```python
from build123d import *

# Parameters (mm, degrees)
F2_DEPTH = 2
F0_R     = 5
F3_DEPTH = 8


with BuildPart() as f2:
    # F1 (on Top) → F2 (new body)
    with BuildSketch(Plane.XY):
        with BuildLine():
            ThreePointArc((13.3352901354, 8.8413820755), (12.5684052501, -9.9012721137), (-5.473909682, -15.0345040754))
            ThreePointArc((-5.473909682, -15.0345040754), (-8.2417855801, -14.8458488198), (-10.6841578939, -16.1617307572))
            ThreePointArc((-10.6841578939, -16.1617307572), (-6.49143908, -46.9599083827), (21.8114936554, -34.112705003))
            Line((21.8114936554, -34.112705003), (25.1481622756, -18.7513405658))
            ThreePointArc((25.1481622756, -18.7513405658), (25.3446435428, -18.0783456566), (25.6333270757, -17.4394490656))
            ThreePointArc((25.6333270757, -17.4394490656), (27.3258914034, -0.6237467424), (16.5919494859, 12.4305670861))
            ThreePointArc((16.5919494859, 12.4305670861), (13.5674787289, 11.902767988), (13.3352901354, 8.8413820755))
        make_face()
    extrude(amount=-F2_DEPTH)

    # F0 (on Top) → F3 (join)
    with BuildSketch(Plane.XY):
        with BuildLine():
            ThreePointArc((9.3589739054, -12.9772727273), (2.1980630587, -15.8482970312), (-5.473909682, -15.0345040754))
            ThreePointArc((-5.473909682, -15.0345040754), (-8.2417855801, -14.8458488198), (-10.6841578939, -16.1617307572))
            ThreePointArc((-10.6841578939, -16.1617307572), (-6.49143908, -46.9599083827), (21.8114936554, -34.112705003))
            Line((21.8114936554, -34.112705003), (25.1481622756, -18.7513405658))
            ThreePointArc((25.1481622756, -18.7513405658), (25.3446435428, -18.0783456566), (25.6333270757, -17.4394490656))
            ThreePointArc((25.6333270757, -17.4394490656), (27.3258914034, -0.6237467424), (16.5919494859, 12.4305670861))
            ThreePointArc((16.5919494859, 12.4305670861), (13.5674787289, 11.902767988), (13.3352901354, 8.8413820755))
            ThreePointArc((13.3352901354, 8.8413820755), (15.9404716471, -1.3788994408), (11.6189500386, -11))
            ThreePointArc((11.6189500386, -11), (14.6969384567, -28.3245553203), (0, -38))
            ThreePointArc((0, -38), (-4.6636895265, -23.5), (7.5784954806, -32.5625))
            ThreePointArc((7.5784954806, -32.5625), (12.9466114923, -23.1769668084), (9.3589739054, -12.9772727273))
        make_face()
        with Locations((0, -30)):
            Circle(F0_R)
    extrude(amount=F3_DEPTH)


solid = f2.part
```
Input: part model. Units: mm. Frame: model coordinates. A direction names the side the tool comes from. Round coordinates to 2 decimals unless told otherwise and drop trailing zeros. Write each loop counter-clockwise with the first axis right and the second up, starting at its lowest first coordinate (ties: lowest second). Pieces come first, ordered by that corner, then holes. Notation, with made-up numbers: (32.25, 68.5) - (77.25, 68.5) arc R18 cw to (77.25, 77.5) - close; hole circle Ø5 at (-27.75, 4). An arc over 180 degrees is marked (long way). Write item = value, one per line.
(1) Access query for faces 5 (the cylindrical face through (-6.93, -46.71, 2.93)), 6 (the cylindrical face through (14.8, -28.08, 3.94)). Directions: +Z, -Z, +X, -X, +Y, -Y. A direction counts if a zero-diameter tool reaches every point of the face in a straight line with its end or side. Return the directions, or none.
Geometry check:
face_5 = +Z, -Z
face_6 = +Z
(2) Material intervals for probe 1 along Y at (x, z) = (-2.5, 6); probe 2 along X at (y, z) = (-24, 3.75); probe 3 along Y at (x, z) = (-1, 5.75), sorted ascending.
Geometry check:
probe_1 = -48.61 to -37.6, -34.33 to -25.67, -22.4 to -15.8
probe_2 = -15.55 to -5.29, 5.29 to 12.85, 15.87 to 24.01
probe_3 = -48.98 to -37.94, -34.9 to -25.1, -22.06 to -15.97
(3) Section query C-C on y = -30. Output: boundary loops of the cut face in (x, z).
Geometry check:
outline = (-16.5, -2) - (22.7, -2) - (22.7, 8) - (13.86, 8) - (13.86, 0) - (10.25, 0) - (10.25, 8) - (8, 8) - (8, 0) - (5, 0) - (5, 8) - (-5, 8) - (-5, 0) - (-8, 0) - (-8, 8) - (-16.5, 8) - close
(4) Section query A-A on z = -0.75. Output: boundary loops of the cut face in (x, y), then the cut area to 3 significant figures.
Geometry check:
outline = (-10.68, -16.16) arc R19.38 ccw (long way) to (21.81, -34.11) - (25.15, -18.75) arc R5 cw to (25.63, -17.44) arc R22 ccw to (16.59, 12.43) arc R2.5 ccw to (13.34, 8.84) arc R16 cw to (-5.47, -15.03) arc R5 ccw to start
area = 1,490 mm^2
(5) Contact query for flat-ended pins moving along their axis: pin 1 Ø1.5 at (x, z) = (-7, 0) entering from +Y; pin 2 Ø2 at (x, z) = (-3, 0) entering from +Y; pin 3 Ø1.5 at (x, z) = (-9, 2) entering from +Y. Output: stop coordinate, or through.
Geometry check:
pin_1 = -14.73
pin_2 = -15.49
pin_3 = -14.85
(6) Pull-direction query (Y, two-part tool) for faces 1 (the cylindrical face through (-1.08, -34.88, 3.94)), 2 (the cylindrical face through (27.395, -0.857, 2.93)), 3 (the flat face through (11, -25, 8)), 4 (the cylindrical face through (12.93, -23.33, 3.94)); classes: +Y half, -Y half, draft (parallel to the pull), parting line (faces both ways), or undercut.
Geometry check:
face_1 = undercut
face_2 = parting line
face_3 = draft
face_4 = undercut
(7) Section query D-D on x = -9.5. Output: boundary loops of the cut face in (y, z).
Geometry check:
outline = (-44.91, -2) - (-15.3, -2) - (-15.3, 8) - (-44.91, 8) - close
(8) Section query B-B on x = 1. Output: boundary loops of the cut face in (y, z).
Geometry check:
outline = (-49.28, -2) - (-15.97, -2) - (-15.97, 8) - (-22.06, 8) - (-22.06, 0) - (-25.1, 0) - (-25.1, 8) - (-34.9, 8) - (-34.9, 0) - (-37.97, 0) - (-37.97, 8) - (-49.28, 8) - close
